Work out the finished part from the listing and answer in its coordinate system (mm). Round coordinates to 2 decimals unless told otherwise and drop trailing zeros. Order: outer loops, then holes, each group sorted by start corner. A loop starts at its lowest first (then second) coordinate and runs counter-clockwise, first axis right, second up.
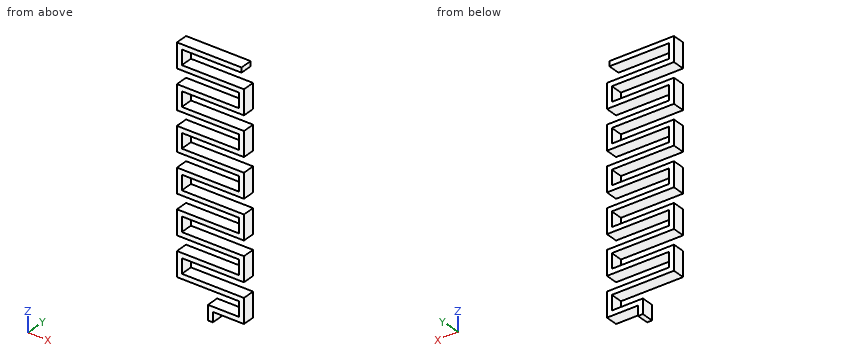
from build123d import *

# Parameters (mm, degrees)
EXTRUDE_THIN1_DEPTH = 5


with BuildPart() as part:
    # Sketch1 → Extrude-Thin1 (new body)
    with BuildSketch(Plane(origin=(0, 0, 0), x_dir=(1, 0, 0), z_dir=(0, 1, 0))):
        Polygon((-1, 0), (-1, -6), (11.7, -6), (11.7, -12), (-13.7, -12), (-13.7, -22), (11.7, -22), (11.7, -28), (-13.7, -28), (-13.7, -38), (11.7, -38), (11.7, -44), (-13.7, -44), (-13.7, -54), (11.7, -54), (11.7, -60), (-13.7, -60), (-13.7, -70), (11.7, -70), (11.7, -76), (-13.7, -76), (-13.7, -86), (11.7, -86), (11.7, -92), (-13.7, -92), (-13.7, -102), (12.7, -102), (12.7, -100), (-11.7, -100), (-11.7, -94), (13.7, -94), (13.7, -84), (-11.7, -84), (-11.7, -78), (13.7, -78), (13.7, -68), (-11.7, -68), (-11.7, -62), (13.7, -62), (13.7, -52), (-11.7, -52), (-11.7, -46), (13.7, -46), (13.7, -36), (-11.7, -36), (-11.7, -30), (13.7, -30), (13.7, -20), (-11.7, -20), (-11.7, -14), (13.7, -14), (13.7, -4), (1, -4), (1, 0), align=None)
    extrude(amount=EXTRUDE_THIN1_DEPTH)


solid = part.part
Item 1: Find the intervals of material crossed by line 1 along Z through (x, y) = (-12.25, 2.3); line 2 along X through (y, z) = (1.75, 74.5); line 3 along X through (y, z) = (1.3, 66.5), in increasing order.
Item 2: Given pin 1 (2.5 mm diameter, centred on x = 1, y = 3, fed in from -Z); pin 2 (2.5 mm diameter, centred on x = -6, y = 3.5, fed in from -Z); pin 3 (2.5 mm diameter, centred on y = 2, z = 1.5, fed in from -X); pin 4 (2.5 mm diameter, centred on y = 2.5, z = 97.5, fed in from +X), each flat-ended and moving along its own axis, determine where each tip first touches the part or whether it passes through.
Item 3: Find section C-C (z = 83). Write down the section's boundary in (x, y).
Item 4: Find section A-A (x = 6.75). State how many separate pieces and enclosed holes the cut face has, plus the area to 3 significant figures.
Model answer:
1. line 1: z = 12 to 22, 28 to 38, 44 to 54, 60 to 70, 76 to 86, 92 to 102
1. line 2: x = 11.7 to 13.7
1. line 3: x = -13.7 to -11.7
2. pin 1: stops at z = 0
2. pin 2: stops at z = 12
2. pin 3: stops at x = -1
2. pin 4: stops at x = -11.7
3. outline: (-13.7, 0) - (-11.7, 0) - (-11.7, 5) - (-13.7, 5) - close
4. separate pieces: 13
4. enclosed holes: 0
4. area: 130 mm2
